Here's how the part is built. I have some questions about the finished solid (model axes, mm). Face numbers are marked on the shaded views. A direction names the side the tool comes from. Round coordinates to 2 decimals unless told otherwise and drop trailing zeros. Loops run counter-clockwise (first coordinate to the right, second up) from the corner with the lowest first, then second, coordinate; pieces in that order, holes last. Notation, with made-up numbers: M 86.5,3 L 95.5,3 A24 ccw 95.5,42 Z; hole C -28.5,80.25 d4. An arc over 180 degrees is marked long. Put each result on its own line as item: value. Start each with the question number.
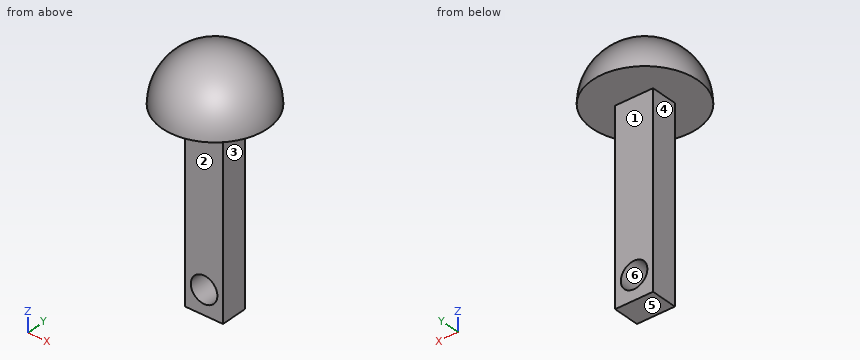
```python
from build123d import *

# Parameters (mm, degrees)
F0_R          = 3.5
F1_DEPTH      = 3.5
F2_ANGLE_BACK = 90
F2_ANGLE      = 180


# Not quite as in the source:
# - a feature of the source that left no trace in its solid (it failed there, or was rolled back) is left out


with BuildPart() as f1:
    # F0 (on Front) → F1 (new body, symmetric)
    with BuildSketch(Plane.XZ):
        with BuildLine():
            ThreePointArc((-4.4455649331, -9.5285820105), (-9.4455649331, -10.4578883784), (-14.4455649331, -9.5285820105))
            Line((-14.4455649331, -9.5285820105), (-14.4455649331, -46.5423427522))
            Line((-14.4455649331, -46.5423427522), (-4.4455649331, -46.5423427522))
            Line((-4.4455649331, -46.5423427522), (-4.4455649331, -9.5285820105))
        make_face()
        with Locations((-9.4455649331, -40.2793101966)):
            Circle(F0_R, mode=Mode.SUBTRACT)
        with BuildLine():
            Line((-4.4455649331, 3.4576572478), (-14.4455649331, 3.4576572478))
            Line((-14.4455649331, 3.4576572478), (-14.4455649331, -9.5285820105))
            ThreePointArc((-14.4455649331, -9.5285820105), (-9.4455649331, -10.4578883784), (-4.4455649331, -9.5285820105))
            Line((-4.4455649331, -9.5285820105), (-4.4455649331, 3.4576572478))
        make_face()
    extrude(amount=F1_DEPTH, both=True)

    # F0 (on Front) → F2 (revolve)
    with BuildSketch(Plane.XZ, mode=Mode.PRIVATE) as f2_sk:
        with BuildLine():
            Line((-23.3611105593, 3.4576572478), (-14.4455649331, 3.4576572478))
            Line((-14.4455649331, 3.4576572478), (-4.4455649331, 3.4576572478))
            Line((-4.4455649331, 3.4576572478), (4.469980693, 3.4576572478))
            ThreePointArc((4.469980693, 3.4576572478), (-9.4455649331, 17.3732028739), (-23.3611105593, 3.4576572478))
        make_face()
    revolve(f2_sk.sketch.rotate(Axis((-13.6577822268, 0, 3.4576572478), (-1, 0, 0)), -F2_ANGLE_BACK), axis=Axis((-13.6577822268, 0, 3.4576572478), (-1, 0, 0)), revolution_arc=F2_ANGLE)


solid = f1.part
```
1) If I drill on probe 1 along X at (y, z) = (-0.5, -18); probe 2 along Y at (x, z) = (-7, -4.5); probe 3 along Z at (x, y) = (-7.25, 1.25), over which ranges is the centre line in solid material (lowest first)? Write a range as from..to.
2) I'm going to push flat-ended pins straight in: P1, Ø6, axis at x = -0.5, y = -9, coming from the +Z side; P2, Ø3, axis at x = -7.5, z = -14, coming from the +Y side; P3, Ø5, axis at x = -17.5, y = 8.5, coming from the -Z side. Where does each tip first touch, or does it pass through?
3) Suppose I cut it at A-A (z = -38). Write out the boundary of the cut face in (x, y), plus the area to 3 significant figures.
4) On a 3-axis mill with a long thin cutter (end or side, diameter ignored), from which of +Z, -Z, +X, -X, +Y, -Y can I reach the whole of each face in a straight line? I mean the marked faces 1 and 2. Say none if no direction works.
5) Suppose I cut it at D-D (z = 1). Write out the boundary of the cut face in (x, y), plus the area to 3 significant figures.
6) Suppose I cut it at C-C (x = -8.75). Write out the boundary of the cut face in (y, z), plus the area to 3 significant figures.
7) Suppose I cut it at B-B (y = 1.5). Write out the boundary of the cut face in (x, z).
8) If we mould it in two halves opening along X, with no side actions, what happens to the marked faces 3, 4, 5 and 6? For each: pulls with the +X half, pulls with the -X half, needs draft (parallel to the pull), parting line crosses it, or undercut.
Results are:
1. probe 1: -14.45..-4.45
1. probe 2: -3.5..3.5
1. probe 3: -46.54..-43.01, -37.55..17.14
2. P1: z = 13.45
2. P2: y = 3.5
2. P3: z = 3.46
3. outline: M -14.45,-3.5 L -12.1,-3.5 L -12.1,3.5 L -14.45,3.5 Z; M -6.79,-3.5 L -4.45,-3.5 L -4.45,3.5 L -6.79,3.5 Z
3. area: 32.8 mm²
4. face 1: -Z, +X, -X, +Y
4. face 2: -Z, +X, -X, -Y
5. outline: M -14.45,-3.5 L -4.45,-3.5 L -4.45,3.5 L -14.45,3.5 Z
5. area: 70.0 mm²
6. outline: M -13.9,3.46 L -3.5,3.46 L -3.5,-36.85 L 3.5,-36.85 L 3.5,3.46 L 13.9,3.46 A13.9 ccw Z; M -3.5,-46.54 L 3.5,-46.54 L 3.5,-43.71 L -3.5,-43.71 Z
6. area: 605 mm²
7. outline: M -23.28,3.46 L -14.45,3.46 L -14.45,-46.54 L -4.45,-46.54 L -4.45,3.46 L 4.39,3.46 A13.83 ccw Z; hole C -9.45,-40.28 d7
8. face 3: pulls with the +X half
8. face 4: pulls with the -X half
8. face 5: needs draft
8. face 6: undercut
